Check sheet for the modelled part. Datum: model origin and axes. Units: mm. A direction names the side the tool comes from. Give positions to 0.01 mm unless a question says otherwise; leave off trailing zeros. Order: outer loops, then holes, each group sorted by start corner. A loop starts at its lowest first (then second) coordinate and runs counter-clockwise, first axis right, second up. Notation, with made-up numbers: (82.5, 13.5) -> (137.5, 13.5) arc R25 ccw to (137.5, 42.5) -> close; hole circle Ø10 at (25.5, 64). An arc over 180 degrees is marked (long way). Write each question's results on one line, items separated by ' | '.
from build123d import *

# Parameters (mm, degrees)
SKETCH_1_W          = 105
SKETCH_1_H          = 105
SKETCH_1_W_2        = 71
SKETCH_1_H_2        = 71
EXTRUDE_1_DEPTH     = 3
SKETCH_2_W          = 77
SKETCH_2_H          = 77
SKETCH_2_W_2        = 71
SKETCH_2_H_2        = 71
EXTRUDE_2_DEPTH     = 7
CHAMFER_1_SIZE      = 1
SKETCH_4_R          = 2.25
CUT_EXTRUDE_1_DEPTH = 4


with BuildPart() as part:
    # Эскиз1 → Бобышка-Вытянуть1 (new body)
    with BuildSketch(Plane.XY):
        with Locations((35.5, 35.5)):
            Rectangle(SKETCH_1_W, SKETCH_1_H)
        with Locations((35.5, 35.5)):
            Rectangle(SKETCH_1_W_2, SKETCH_1_H_2, mode=Mode.SUBTRACT)
    extrude(amount=EXTRUDE_1_DEPTH)

    # Эскиз2 → Бобышка-Вытянуть2 (add)
    with BuildSketch(Plane.XY.offset(3)):
        with Locations((35.5, 35.5)):
            Rectangle(SKETCH_2_W, SKETCH_2_H)
        with Locations((35.5, 35.5)):
            Rectangle(SKETCH_2_W_2, SKETCH_2_H_2, mode=Mode.SUBTRACT)
    extrude(amount=EXTRUDE_2_DEPTH)

    # Фаска1
    chamfer_1_edges = [part.edges().sort_by_distance(p)[0] for p in [
        (-3, 35.5, 10),
        (35.5, -3, 10),
        (74, 35.5, 10),
        (35.5, 74, 10),
        (-3, 35.5, 3),
        (35.5, -3, 3),
        (74, 35.5, 3),
        (35.5, 74, 3),
    ]]
    chamfer(chamfer_1_edges, length=CHAMFER_1_SIZE)

    # Эскиз4 → Вырез-Вытянуть1 (cut, through all)
    with BuildSketch(Plane.XY.offset(3)):
        with Locations((-11, 82)):
            Circle(SKETCH_4_R)
        with Locations((82, 82)):
            Circle(SKETCH_4_R)
        with Locations((82, -11)):
            Circle(SKETCH_4_R)
        with Locations((-11, -11)):
            Circle(SKETCH_4_R)
    extrude(amount=-CUT_EXTRUDE_1_DEPTH, mode=Mode.SUBTRACT)


solid = part.part
1. Mould release check, pull along X, two halves, no side actions. Record for faces 6 (the flat face through (-17, 35, 1)), 7 (the flat face through (35, 71, 5)), 8 (the flat face through (-0.2, 36.2, 0)): +X half, -X half, draft (parallel to the pull), parting line (faces both ways), or undercut.
Verdict:
face 6: -X half | face 7: undercut | face 8: draft
2. Section check C-C on z = 6. Record the cut outline in (x, y).
Verdict:
outline: (-3, -3) -> (74, -3) -> (74, 74) -> (-3, 74) -> close; hole (0, 0) -> (71, 0) -> (71, 71) -> (0, 71) -> close
3. Access from +Z, -Z, +X, -X, +Y, -Y to the whole of each face (thin tool, end or side, straight path). Record for faces 1 (the flat face through (-3, 35, 6)), 2 (the flat face through (35, -3, 6)), 3 (the flat face through (-8, 40, 3)), 4 (the flat face through (35, 74, 6)), 5 (the flat face through (0, 35, 5)).
Verdict:
face 1: +Z, -X, +Y, -Y | face 2: +Z, +X, -X, -Y | face 3: +Z | face 4: +Z, +X, -X, +Y | face 5: +Z, -Z
4. Material ranges on probe 1 along Y at (x, z) = (-11, 1.15); probe 2 along Y at (x, z) = (64, 5); probe 3 along X at (y, z) = (46, 2.75), recorded low to high. Write a range as from..to.
Verdict:
probe 1: y = -17..-13.25, -8.75..79.75, 84.25..88 | probe 2: y = -3..0, 71..74 | probe 3: x = -17..0, 71..88
5. Section check D-D on x = 38.5. Record the cut outline in (y, z).
Verdict:
outline: (-17, 0) -> (0, 0) -> (0, 10) -> (-2, 10) -> (-3, 9) -> (-3, 4) -> (-4, 3) -> (-17, 3) -> close; (71, 0) -> (88, 0) -> (88, 3) -> (75, 3) -> (74, 4) -> (74, 9) -> (73, 10) -> (71, 10) -> close
6. Gauge pin test, flat ends, axial feed: pin 1 Ø2.5 at (x, z) = (18.5, 7) entering from -Y; pin 2 Ø3 at (x, z) = (19.5, 8.5) entering from +Y; pin 3 Ø5.5 at (x, z) = (21.5, 6) entering from +Y. Record the tip position at first contact, or that the pin passes through.
Verdict:
pin 1: stops at y = -3 | pin 2: stops at y = 74 | pin 3: stops at y = 74.75
7. Section check A-A on x = 82. Record the cut outline in (y, z), then the cut area to 3 significant figures.
Verdict:
outline: (-17, 0) -> (-13.25, 0) -> (-13.25, 3) -> (-17, 3) -> close; (-8.75, 0) -> (79.75, 0) -> (79.75, 3) -> (-8.75, 3) -> close; (84.25, 0) -> (88, 0) -> (88, 3) -> (84.25, 3) -> close | area: 288 mm^2
